Source: three-view drawing plus pictorial views. Frame: mm from the lowest corner of the part. Give positions to 0.01 mm unless a question says otherwise; leave off trailing zeros. Order: outer loops, then holes, each group sorted by start corner. A loop starts at its lowest first (then second) coordinate and runs counter-clockwise, first axis right, second up. Notation, with made-up numbers: (0.5, -21) - (52.5, -21) arc R11 ccw to (52.5, -14) - close; hole circle Ø7 at (-20.5, -18). An arc over 180 degrees is marked (long way). Use CSV: the item, a comma, the result in double quotes.
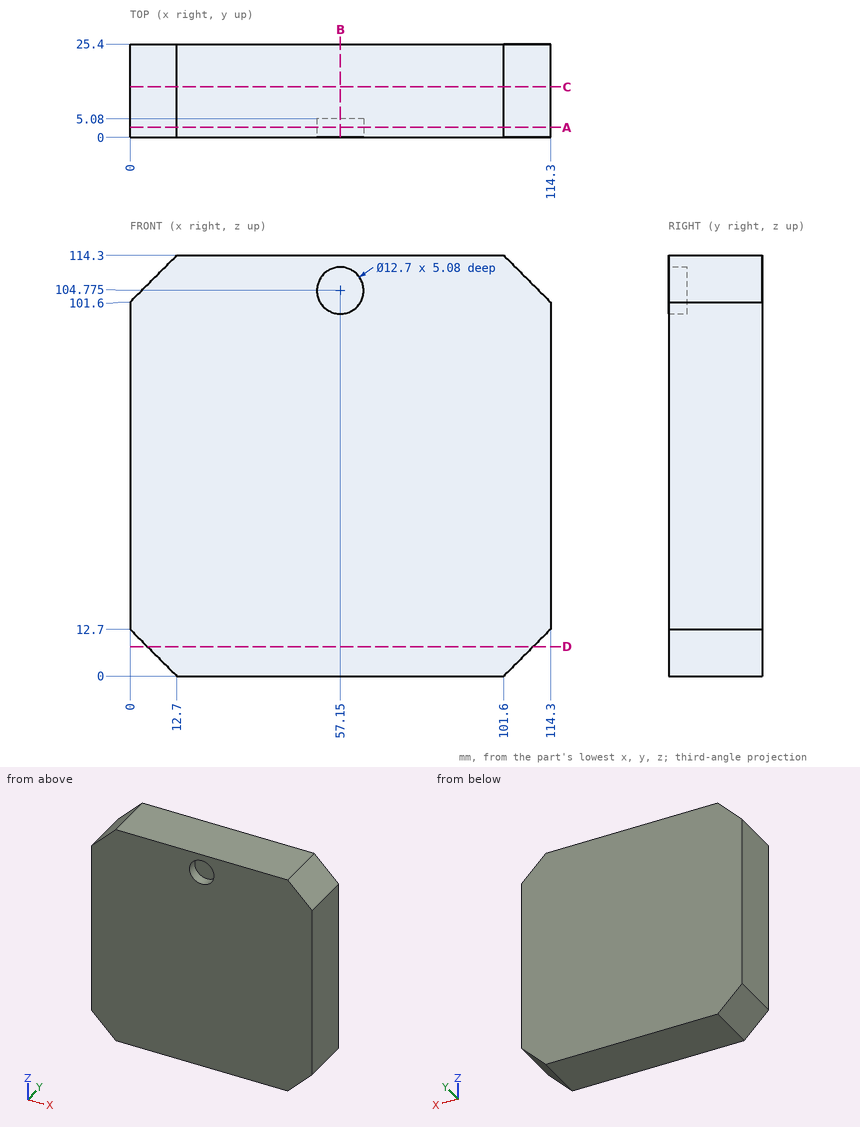
Item 1: Material intervals for line 1 (Y direction, x = 51.5, z = 107); line 2 (X direction, y = 23.5, z = 102); line 3 (X direction, y = 2.75, z = 10), sorted ascending. Write a range as from..to.
Filled in:
line 1,"y = 5.08..25.4"
line 2,"x = 0.4..113.9"
line 3,"x = 2.7..111.6"
Item 2: Section B-B on x = 57.15. Return the cut outline in (y, z) (3 decimals), then the cut area to 3 significant figures.
Filled in:
outline,"(0, 0) - (25.4, 0) - (25.4, 114.3) - (0, 114.3) - (0, 111.125) - (5.08, 111.125) - (5.08, 98.425) - (0, 98.425) - close"
area,"2,840 mm2"
Item 3: Section C-C on y = 13.75. Return the cut outline in (x, z).
Filled in:
outline,"(0, 12.7) - (12.7, 0) - (101.6, 0) - (114.3, 12.7) - (114.3, 101.6) - (101.6, 114.3) - (12.7, 114.3) - (0, 101.6) - close"
Item 4: Section D-D on z = 8. Return the cut outline in (x, y), then the cut area to 3 significant figures.
Filled in:
outline,"(4.7, 0) - (109.6, 0) - (109.6, 25.4) - (4.7, 25.4) - close"
area,"2,660 mm2"
Item 5: Section A-A on y = 2.75. Return the cut outline in (x, z) (3 decimals).
Filled in:
outline,"(0, 12.7) - (12.7, 0) - (101.6, 0) - (114.3, 12.7) - (114.3, 101.6) - (101.6, 114.3) - (12.7, 114.3) - (0, 101.6) - close; hole circle Ø12.7 at (57.15, 104.775)"
